```python
from build123d import *

# Parameters (mm, degrees)
F0_R     = 41.283665
F1_DEPTH = 76.2
F2_SIZE  = 5.08
F3_T     = -2.54


with BuildPart() as f1:
    # F0 (on Top) → F1 (new body)
    with BuildSketch(Plane.XY):
        Circle(F0_R)
    extrude(amount=F1_DEPTH)

    # F2
    f2_edges = [f1.edges().sort_by_distance(p)[0] for p in [
        (-41.283665, 0, 76.2),
    ]]
    chamfer(f2_edges, length=F2_SIZE)

    # F3
    f3_openings = [f1.faces().sort_by_distance(p)[0] for p in [
        (0, 0, 0),
    ]]
    offset(amount=F3_T, openings=f3_openings)


solid = f1.part
```
Can you work these out from the model? Positions are in its coordinate system, mm. A direction names the side the tool comes from. Round coordinates to 2 decimals unless told otherwise and drop trailing zeros. Loops run counter-clockwise (first coordinate to the right, second up) from the corner with the lowest first, then second, coordinate; pieces in that order, holes last. Notation, with made-up numbers: M -20,-5.75 L 21,-5.75 A30 cw 21,31.25 Z; hole C -24.75,34.5 d10. An arc over 180 degrees is marked long. Write item = value, one per line. Start each with the question number.
(1) Which directions (+Z, -Z, +X, -X, +Y, -Y) give clear straight access to the entire face, cutting with the end or side of a thin tool? Please do faces 1 (the face through (0, 0, 73.66)), 2 (the face through (12, 37, 0)).
(2) I'm going to push flat-ended pins straight in: P1, Ø8, axis at y = -9, z = 29, coming from the -X side; P2, Ø4, axis at x = 12, z = 44.5, coming from the -Y side; P3, Ø3, axis at x = -12, z = 12.5, coming from the -Y side; P4, Ø12, axis at y = 1.5, z = 45, coming from the -X side. Where does each tip first touch, or does it pass through?
(3) I need wall thicknesses on line 1 along Y through (x, z) = (0, 56.5); line 2 along Y through (x, z) = (20.5, 55); line 3 along X through (y, z) = (-35, 24). Which ranges of each line are inside material? Lowest first, please.
(4) Suppose I cut it at B-B on z = 50. Write out the boundary of the cut face in (x, y), plus the area to 3 significant figures.
(5) If we mould it in two halves opening along X, with no side actions, what happens to faces 3 (the face through (-38.706, 1.703, 34.543)), 4 (the face through (-1, 1, 76.2)), 5 (the face through (34.77, 10.95, 75.95))? For each: released by +X, released by -X, zero draft, split by the parting line, or undercut.
(6) Suppose I cut it at A-A on x = 0. Write out the boundary of the cut face in (y, z).
Answer block:
q1.face_1 = -Z
q1.face_2 = -Z, +X, -X, +Y, -Y
q2.P1 = -40.98
q2.P2 = -40.05
q2.P3 = -39.93
q2.P4 = -41.28
q3.line_1 = -41.28 to -38.74, 38.74 to 41.28
q3.line_2 = -35.83 to -32.88, 32.88 to 35.83
q3.line_3 = -21.89 to -16.62, 16.62 to 21.89
q4.outline = C 0,0 d82.57; hole C 0,0 d77.49
q4.area = 639 mm²
q5.face_3 = undercut
q5.face_4 = zero draft
q5.face_5 = split by the parting line
q6.outline = M -41.28,0 L -38.74,0 L -38.74,70.07 L -35.15,73.66 L 35.15,73.66 L 38.74,70.07 L 38.74,0 L 41.28,0 L 41.28,71.12 L 36.2,76.2 L -36.2,76.2 L -41.28,71.12 Z
